```python
from build123d import *

# Parameters (mm, degrees)
CROQUIS1_R                   = 9
CROQUIS1_R_2                 = 1.5
SALIENTE_EXTRUIR1_DEPTH      = 15
SALIENTE_EXTRUIR1_DEPTH_BACK = 8
CROQUIS2_R                   = 9
CROQUIS2_R_2                 = 4
SALIENTE_EXTRUIR4_DEPTH      = 20
CROQUIS7_R                   = 4
CORTAR_EXTRUIR1_DEPTH        = 20
CROQUIS8_R                   = 1.5
CORTAR_EXTRUIR2_DEPTH        = 15
CROQUIS9_R                   = 1.4
CORTAR_EXTRUIR3_DEPTH        = 19
CROQUIS10_R                  = 1.4
CORTAR_EXTRUIR4_DEPTH        = 1
CORTAR_EXTRUIR4_DEPTH_BACK   = 33.0000001


with BuildPart() as part:
    # Croquis1 → Saliente-Extruir1 (new body, two sides)
    with BuildSketch(Plane.XY) as saliente_extruir1_sk:
        Circle(CROQUIS1_R)
        Circle(CROQUIS1_R_2, mode=Mode.SUBTRACT)
    extrude(amount=SALIENTE_EXTRUIR1_DEPTH)
    extrude(saliente_extruir1_sk.sketch, amount=-SALIENTE_EXTRUIR1_DEPTH_BACK)

    # Croquis2 → Saliente-Extruir4 (add)
    with BuildSketch(Plane(origin=(0, 0, 0), x_dir=(1, 0, 0), z_dir=(0, 1, 0))):
        with Locations((0, 8)):
            Circle(CROQUIS2_R)
        with Locations((0, 8)):
            Circle(CROQUIS2_R_2, mode=Mode.SUBTRACT)
    extrude(amount=SALIENTE_EXTRUIR4_DEPTH)

    # Croquis6 → Revolución4 (revolve)
    with BuildSketch(Plane(origin=(0, 0, -8), x_dir=(-1, 0, 0), z_dir=(0, 0, -1))):
        with BuildLine():
            Line((0, 0), (0, -9))
            ThreePointArc((0, -9), (-6.363961031, -6.363961031), (-9, 0))
            Line((-9, 0), (0, 0))
        make_face()
    revolve(axis=Axis((0, 0, -8), (0, -1, 0)))

    # Croquis7 → Cortar-Extruir1 (cut)
    with BuildSketch(Plane(origin=(0, 20, 0), x_dir=(1, 0, 0), z_dir=(0, 1, 0))):
        with Locations((0, 8)):
            Circle(CROQUIS7_R)
    extrude(amount=-CORTAR_EXTRUIR1_DEPTH, mode=Mode.SUBTRACT)

    # Croquis8 → Cortar-Extruir2 (cut)
    with BuildSketch(Plane.XY.offset(15)):
        Circle(CROQUIS8_R)
    extrude(amount=-CORTAR_EXTRUIR2_DEPTH, mode=Mode.SUBTRACT)

    # Croquis9 → Cortar-Extruir3 (cut, through all)
    with BuildSketch(Plane.ZY.offset(9)):
        with Locations((8, 0)):
            Circle(CROQUIS9_R)
    extrude(amount=-CORTAR_EXTRUIR3_DEPTH, mode=Mode.SUBTRACT)

    # Croquis10 → Cortar-Extruir4 (cut, two sides)
    with BuildSketch(Plane(origin=(0, 0, -17), x_dir=(-1, 0, 0), z_dir=(0, 0, -1))) as cortar_extruir4_sk:
        with Locations((0, 13.459047629)):
            Circle(CROQUIS10_R)
    extrude(amount=CORTAR_EXTRUIR4_DEPTH, mode=Mode.SUBTRACT)
    extrude(cortar_extruir4_sk.sketch, amount=-CORTAR_EXTRUIR4_DEPTH_BACK, mode=Mode.SUBTRACT)


solid = part.part
```
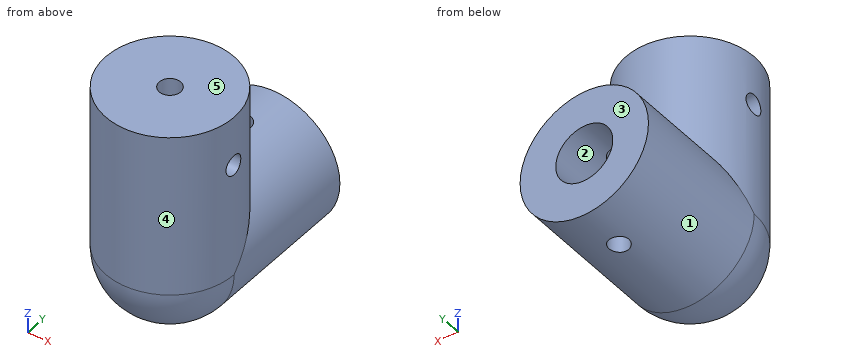
The model under review builds one solid part; all positions refer to its coordinate system, in mm. Face numbers are marked on the shaded views. A direction names the side the tool comes from. Give positions to 0.01 mm unless a question says otherwise; leave off trailing zeros. Write each loop counter-clockwise with the first axis right and the second up, starting at its lowest first coordinate (ties: lowest second). Pieces come first, ordered by that corner, then holes. Notation, with made-up numbers: (-24, 19) -> (-14, 19) arc R11 ccw to (-14, 35) -> close; hole circle Ø8 at (-1.5, 10). An arc over 180 degrees is marked (long way). Answer in a Markdown table with one row per item.
1) Add section B-B on x = 0. State the section outline as (y, z) points.
Worked answers:
| item | result |
|---|---|
| outline | (-9, -8) arc R9 ccw to (0, -17) -> (12.06, -17) -> (12.06, -12) -> (0, -12) -> (0, -4) -> (12.06, -4) -> (12.06, 1) -> (9, 1) -> (9, 15) -> (1.5, 15) -> (1.5, 0) -> (-1.5, 0) -> (-1.5, 15) -> (-9, 15) -> close; (14.86, -17) -> (20, -17) -> (20, -12) -> (14.86, -12) -> close; (14.86, -4) -> (20, -4) -> (20, 1) -> (14.86, 1) -> close |
2) Add section A-A on y = 0.75. State the section outline as (x, z) points, plus the area to 3 significant figures.
Worked answers:
| item | result |
|---|---|
| outline | (-8.97, -7.25) arc R9 ccw (long way) to (8.97, -7.25) -> (8.97, 6.82) -> (1.3, 6.82) -> (1.3, 0) -> (-1.3, 0) -> (-1.3, 6.82) -> (-8.97, 6.82) -> close; (-8.97, 9.18) -> (-1.3, 9.18) -> (-1.3, 15) -> (-8.97, 15) -> close; (1.3, 9.18) -> (8.97, 9.18) -> (8.97, 15) -> (1.3, 15) -> close; hole circle Ø8 at (0, -8) |
| area | 414 mm² |
3) Add section C-C on y = 12.5. State the section outline as (x, z) points.
Worked answers:
| item | result |
|---|---|
| outline | (-1.02, -16.94) -> (-1.02, -11.87) arc R4 cw to (-1.02, -4.13) -> (-1.02, 0.94) arc R9 ccw to start; (1.02, -16.94) arc R9 ccw to (1.02, 0.94) -> (1.02, -4.13) arc R4 cw to (1.02, -11.87) -> close |
4) Add section D-D on z = 8. State the section outline as (x, y) points, plus the area to 3 significant figures.
Worked answers:
| item | result |
|---|---|
| outline | (-8.89, -1.4) arc R9 ccw to (8.89, -1.4) -> (0.54, -1.4) arc R1.5 cw to (-0.54, -1.4) -> close; (-8.89, 1.4) -> (-0.54, 1.4) arc R1.5 cw to (0.54, 1.4) -> (8.89, 1.4) arc R9 ccw to start |
| area | 204 mm² |
5) Clearance check with flat-ended pins moving along their axes: P1, Ø5, axis at x = -7, z = -6, coming from the -Y side; P2, Ø2.5, axis at x = 0, y = 0, coming from the +Z side; P3, Ø1, axis at x = 6.5, z = -8.5, coming from the -Y side; P4, Ø1.7, axis at y = 0, z = 8, coming from the +X side. State where each tip first meets the part, or that it passes through.
Worked answers:
| item | result |
|---|---|
| P1 | y = -7.79 |
| P2 | z = 0 |
| P3 | y = -6.69 |
| P4 | through |
6) Tool access review of the marked faces 4 and 5: name each direction out of +Z, -Z, +X, -X, +Y, -Y from which nothing blocks a thin tool from reaching the whole face with its end or side.
Worked answers:
| item | result |
|---|---|
| face 4 | +Z |
| face 5 | +Z, +X, -X, +Y, -Y |
7) Mouldability with a two-part tool opening along Z and no side actions: class the marked faces 1, 2 and 3 as +Z half, -Z half, draft (parallel to the pull), parting line (faces both ways), or undercut.
Worked answers:
| item | result |
|---|---|
| face 1 | parting line |
| face 2 | undercut |
| face 3 | draft |
8) For L1, parallel to Y at x = 0, z = 0.75; L2, parallel to Z at x = -1.75, y = 6; L3, parallel to Z at x = 7.25, y = 0, list the stretches that pass through material, from the lowest coordinate up. Write a range as [from, to].
Worked answers:
| item | result |
|---|---|
| L1 | [-9, -1.5], [1.5, 12.06], [14.86, 20] |
| L2 | [-16.83, -11.6], [-4.4, 15] |
| L3 | [-13.33, 6.6], [9.4, 15] |
